Read the model definition and answer for the solid it produces. Units are mm, in the model's axes. Face numbers are marked on the shaded views. A direction names the side the tool comes from. Round coordinates to 2 decimals unless told otherwise and drop trailing zeros. Write each loop counter-clockwise with the first axis right and the second up, starting at its lowest first coordinate (ties: lowest second). Pieces come first, ordered by that corner, then holes. Notation, with made-up numbers: (74.5, 73.25) -> (110.5, 73.25) arc R20 cw to (110.5, 90.25) -> close; hole circle Ø7 at (55, 61). An arc over 180 degrees is marked (long way). Return JSON: item names as keys, results as strings.
from build123d import *

# Parameters (mm, degrees)
SKETCH013_R     = 3.630449
POCKET007_DEPTH = 8.001
CHAMFER_SIZE    = 0.2


with BuildPart() as part:
    # Sketch012 → Revolution001 (revolve)
    with BuildSketch(Plane.XZ):
        Polygon((1.4224, 5), (1.4224, 1.821223), (0, 1), (0, -3), (0.9224, -3), (1.4224, -2.5), (1.4224, 0), (2.1, 0), (3.1, 0.57735), (3.1, 4.42265), (2.1, 5), align=None)
    revolve(axis=Axis((0, 0, 0), (0, 0, 1)))

    # Sketch013 (on Face10 of Revolution001) → Pocket007 (cut, through all)
    with BuildSketch(Plane(origin=(0, 0, 5), x_dir=(-1, 0, 0), z_dir=(0, 0, 1))):
        Circle(SKETCH013_R)
        Polygon((2.424871, 0), (1.212436, 2.1), (-1.212436, 2.1), (-2.424871, 0), (-1.212436, -2.1), (1.212436, -2.1), align=None, mode=Mode.SUBTRACT)
    extrude(amount=-POCKET007_DEPTH, mode=Mode.SUBTRACT)

    # Chamfer
    chamfer_edges = [part.edges().sort_by_distance(p)[0] for p in [
        (-1.4224, 0, 5),
    ]]
    chamfer(chamfer_edges, length=CHAMFER_SIZE)


with BuildPart() as part_1:
    # Body004 placement: moved
    add(part.part.moved(Location((-12.495, 0, 0.9))))


with BuildPart() as part_2:
    # Clone001 placement: moved
    add(part_1.part.moved(Location((12.495, 0, -0.9))))


with BuildPart() as part_3:
    # Body005 placement: moved
    add(part_2.part.moved(Location((12.495, 0, 0.9))))


solid = part_3.part
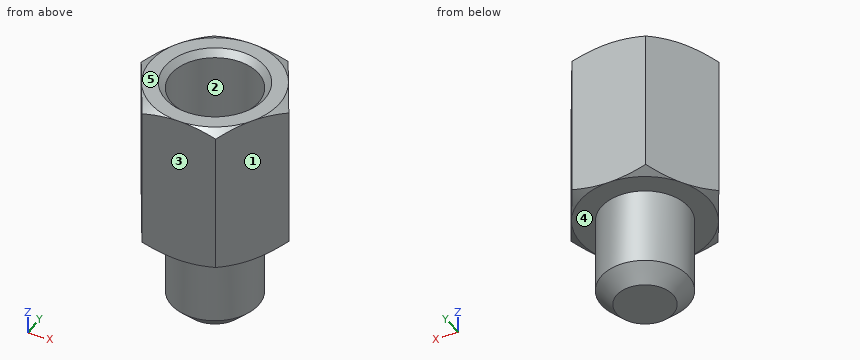
Item 1: Section C-C (z = -1) is taken. Give the vertices of the cut face in (x, y) (3 decimals).
Worked answers:
{"outline": "circle Ø2.845 at (12.495, 0)"}
Item 2: Section B-B (z = 2.5) is taken. Give the vertices of the cut face in (x, y) (3 decimals), then the cut area to 3 significant figures.
Worked answers:
{"outline": "(10.07, 0) -> (11.283, -2.1) -> (13.707, -2.1) -> (14.92, 0) -> (13.707, 2.1) -> (11.283, 2.1) -> close; hole circle Ø2.078 at (12.495, 0)", "area": "11.9 mm2"}
Item 3: Straight lines are drawn through the part: L1, parallel to Z at x = 14.3, y = -0.55; L2, parallel to Y at x = 12.55, z = 2.75; L3, parallel to Y at x = 11.45, z = 5.25. For each, find the intervals that lie inside material, in ascending order. Write a range as [from, to].
Worked answers:
{"L1": "z = [0.9, 5.9]", "L2": "y = [-2.1, -1.42], [1.42, 2.1]", "L3": "y = [-2.1, -0.96], [0.96, 2.1]"}
Item 4: A tool of negligible diameter and unlimited length cuts with its end or side. For the marked faces 4 and 5, from which of +Z, -Z, +X, -X, +Y, -Y can it reach the whole face along a straight path? Write none if from no direction.
Worked answers:
{"face 4": "-Z", "face 5": "+Z, +X, -X, +Y, -Y"}
Item 5: For a pull along X with two mould halves and no side action, classify the marked faces 1, 2 and 3 as released by +X, released by -X, zero draft, split by the parting line, or undercut.
Worked answers:
{"face 1": "released by +X", "face 2": "undercut", "face 3": "zero draft"}
Item 6: Section A-A (z = 4.5) is taken. Give the vertices of the cut face in (x, y) (3 decimals), then the cut area to 3 significant figures.
Worked answers:
{"outline": "(10.07, 0) -> (11.283, -2.1) -> (13.707, -2.1) -> (14.92, 0) -> (13.707, 2.1) -> (11.283, 2.1) -> close; hole circle Ø2.845 at (12.495, 0)", "area": "8.92 mm2"}
Item 7: Flat-ended cylindrical pins translate along their axes: pin 1 (1.7 mm diameter, centred on x = 12.495, y = 0, fed in from +Z); pin 2 (1 mm diameter, centred on y = 1.5, z = 2.5, fed in from -X). Find the tip coordinate at first contact, or state that the pin passes through.
Worked answers:
{"pin 1": "stops at z = 2.39", "pin 2": "stops at x = 10.65"}
